```python
from build123d import *

# Parameters (mm, degrees)
F0_W = 27.4674350193
F0_H = 81.2209066684
F5_R = 1.27


with BuildPart() as f1:
    # F0 (on Front) → F1 (revolve)
    with BuildSketch(Plane.XZ):
        with Locations((-13.7337175096, -0.5906961542)):
            Rectangle(F0_W, F0_H)
    revolve(axis=Axis((0, 0, -0.5906961542), (0, 0, 1)))

    # F0 (on Front) → F2 (revolve)
    with BuildSketch(Plane.XZ):
        with BuildLine():
            Line((-27.4674350193, 40.0197571801), (0, 40.0197571801))
            Line((0, 40.0197571801), (0, 83.1406737302))
            Line((0, 83.1406737302), (-10.1947877868, 83.1406737302))
            add(Edge.make_bspline(
                [(-10.1947877868, 83.1406737302), (-13.0487030437, 62.5508222314), (-28.143446303, 58.3851752324), (-27.4674350193, 40.0197571801)],
                knots=[5.8791278865, 5.8791278865, 5.8791278865, 5.8791278865, 54.3602169565, 54.3602169565, 54.3602169565, 54.3602169565], degree=3))
        make_face()
    revolve(axis=Axis((0, 0, 65.7150976558), (0, 0, 1)))

    # F0 (on Front) → F3 (revolve)
    with BuildSketch(Plane.XZ):
        with BuildLine():
            Line((-10.1947877868, 83.1406737302), (0, 83.1406737302))
            Line((0, 83.1406737302), (0, 91.4104381316))
            Line((0, 91.4104381316), (-9.746512388, 91.4104381316))
            add(Edge.make_bspline(
                [(-9.746512388, 91.4104381316), (-9.6826276693, 88.3759155541), (-9.8487037137, 85.6375312152), (-10.1947877868, 83.1406737302)],
                knots=[0, 0, 0, 0, 5.8791278865, 5.8791278865, 5.8791278865, 5.8791278865], degree=3))
        make_face()
    revolve(axis=Axis((0, 0, 65.7150976558), (0, 0, 1)))

    # F0 (on Front) → F4 (revolve)
    with BuildSketch(Plane.XZ):
        Polygon((-9.746512388, 91.4104381316), (0, 91.4104381316), (0, 95.5453233728), (-12.7, 95.5453233728), (-12.7, 91.4104381316), align=None)
    revolve(axis=Axis((0, 0, 93.4778807522), (0, 0, 1)))

    # F5
    f5_edges = [f1.edges().sort_by_distance(p)[0] for p in [
        (12.7, 0, 91.410438),
        (12.7, 0, 95.545323),
        (27.467435, 0, -41.201149),
    ]]
    fillet(f5_edges, radius=F5_R)


solid = f1.part
```
For this review, take the finished solid that the model builds, in its own axes (mm). A direction names the side the tool comes from. Round coordinates to 2 decimals unless told otherwise and drop trailing zeros. Loops run counter-clockwise (first coordinate to the right, second up) from the corner with the lowest first, then second, coordinate; pieces in that order, holes last.
Q1. Insertion check: pin 1 Ø2 at (x, z) = (12.5, 28) entering from +Y; pin 2 Ø1 at (x, y) = (-18.5, -13.5) entering from +Z; pin 3 Ø1.5 at (y, z) = (-16, 46) entering from +X. Each pin has a flat end and moves straight along its axis. Give the tip position at first contact, or say it passes through.
Result sheet:
pin 1: stops at y = 24.94
pin 2: stops at z = 57.36
pin 3: stops at x = 22.41
Q2. To check wall thickness, follow line 1 along X through (y, z) = (22.5, 8); line 2 along Z through (x, y) = (-14.5, 21); line 3 along Y through (x, z) = (-4.5, 4). State the ranges of each line that lie inside material, in increasing order.
Result sheet:
line 1: x = -15.75 to 15.75
line 2: z = -41.2 to 51.45
line 3: y = -27.1 to 27.1
Q3. Machinability: for faces 1 (the face through (2.75, 12.4, 93.47)), 2 (the face through (-9.3, -3.4, 91.41)), which of the approach directions +Z, -Z, +X, -X, +Y, -Y give a long, thin tool a straight path to every point of the face, cutting with its end or side? Answer none if there is none.
Result sheet:
face 1: +Z
face 2: none
Q4. Add section A-A on z = 4. Write out the cut boundary in (x, y).
Result sheet:
outline: circle Ø54.93 at (0, 0)
